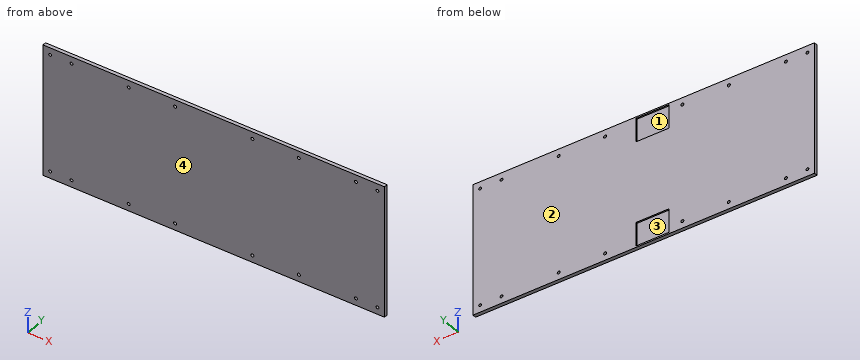
```python
from build123d import *

# Parameters (mm, degrees)
ESQUISSE1_W             = 478.153686012
ESQUISSE1_H             = 188.593708553
ESQUISSE1_R             = 2
BOSS_EXTRU_4_DEPTH      = 5
ESQUISSE2_W             = 35.2
ESQUISSE2_H             = 34
ESQUISSE2_W_2           = 11
ENL_V_MAT_EXTRU_1_DEPTH = 2
ESQUISSE3_R             = 2.1
ENL_V_MAT_EXTRU_2_DEPTH = 10


with BuildPart() as part:
    # Esquisse1 → Boss.-Extru.4 (new body)
    with BuildSketch(Plane(origin=(0, 0, 0), x_dir=(1, 0, 0), z_dir=(0, 1, 0))):
        with Locations((166.159297522, 47.085285911)):
            Rectangle(ESQUISSE1_W, ESQUISSE1_H)
        with Locations(Location((-62.917545484, 131.382140187, 0), (0, 0, 270))):
            Circle(ESQUISSE1_R, mode=Mode.SUBTRACT)
        with Locations(Location((-62.917545484, -37.211568366, 0), (0, 0, 270))):
            Circle(ESQUISSE1_R, mode=Mode.SUBTRACT)
        with Locations(Location((395.236140528, -37.211568366, 0), (0, 0, 270))):
            Circle(ESQUISSE1_R, mode=Mode.SUBTRACT)
        with Locations(Location((395.236140528, 131.382140187, 0), (0, 0, 270))):
            Circle(ESQUISSE1_R, mode=Mode.SUBTRACT)
        with Locations(Location((-32.917545484, -37.211568366, 0), (0, 0, 270))):
            Circle(ESQUISSE1_R, mode=Mode.SUBTRACT)
        with Locations(Location((-32.917545484, 131.382140187, 0), (0, 0, 270))):
            Circle(ESQUISSE1_R, mode=Mode.SUBTRACT)
        with Locations(Location((365.236140528, 131.382140187, 0), (0, 0, 270))):
            Circle(ESQUISSE1_R, mode=Mode.SUBTRACT)
        with Locations(Location((365.236140528, -37.211568366, 0), (0, 0, 270))):
            Circle(ESQUISSE1_R, mode=Mode.SUBTRACT)
    extrude(amount=BOSS_EXTRU_4_DEPTH)

    # Esquisse2 → Enlèv. mat.-Extru.1 (cut)
    with BuildSketch(Plane(origin=(0, 5, 0), x_dir=(1, 0, 0), z_dir=(0, 1, 0))):
        with Locations((148.559297522, 122.382140187)):
            Rectangle(ESQUISSE2_W, ESQUISSE2_H)
        with Locations((171.659297522, 122.382140187)):
            Rectangle(ESQUISSE2_W_2, ESQUISSE2_H)
        with Locations((148.559297522, -28.211568366)):
            Rectangle(ESQUISSE2_W, ESQUISSE2_H)
        with Locations((171.659297522, -28.211568366)):
            Rectangle(ESQUISSE2_W_2, ESQUISSE2_H)
    extrude(amount=-ENL_V_MAT_EXTRU_1_DEPTH, mode=Mode.SUBTRACT)

    # Esquisse3 → Enlèv. mat.-Extru.2 (cut)
    with BuildSketch(Plane(origin=(0, 5, 0), x_dir=(1, 0, 0), z_dir=(0, 1, 0))):
        with Locations(Location((47.082454516, 131.382140187, 0), (0, 0, 270))):
            Circle(ESQUISSE3_R)
        with Locations(Location((47.082454516, -37.211568366, 0), (0, 0, 270))):
            Circle(ESQUISSE3_R)
        with Locations(Location((285.236140528, 131.382140187, 0), (0, 0, 270))):
            Circle(ESQUISSE3_R)
        with Locations(Location((285.236140528, -37.211568366, 0), (0, 0, 270))):
            Circle(ESQUISSE3_R)
        with Locations(Location((220.236140528, 131.382140187, 0), (0, 0, 270))):
            Circle(ESQUISSE3_R)
        with Locations(Location((220.236140528, -37.211568366, 0), (0, 0, 270))):
            Circle(ESQUISSE3_R)
        with Locations(Location((112.082454516, 131.382140187, 0), (0, 0, 270))):
            Circle(ESQUISSE3_R)
        with Locations(Location((112.082454516, -37.211568366, 0), (0, 0, 270))):
            Circle(ESQUISSE3_R)
    extrude(amount=-ENL_V_MAT_EXTRU_2_DEPTH, mode=Mode.SUBTRACT)


solid = part.part
```
Part model, mm, in its own coordinate system. Face numbers are marked on the shaded views. A direction names the side the tool comes from. Round coordinates to 2 decimals unless told otherwise and drop trailing zeros. Write each loop counter-clockwise with the first axis right and the second up, starting at its lowest first coordinate (ties: lowest second). Pieces come first, ordered by that corner, then holes. Notation, with made-up numbers: (32.25, 10.25) -> (45.25, 10.25) arc R13 cw to (45.25, 21.25) -> close; hole circle Ø4 at (47.5, -22). An arc over 180 degrees is marked (long way). Return JSON: item names as keys, results as strings. Group by question number.
Q1. Pin check, flat tip, straight feed: pin 1 (5 mm diameter, centred on x = -62.92, z = -131.38, fed in from +Y). Stop position of the tip, or through.
Q2. Saw through at A-A on x = 138. Write the cut outline in (y, z).
Q3. Which spindle directions (+Z, -Z, +X, -X, +Y, -Y) get a long thin tool onto all of the face, cutting with end or side? Do the marked faces 3 and 4. Say none if no direction does.
Q4. Mould opens along Z. For the marked faces 1 and 2 say: pulls with the +Z half, pulls with the -Z half, needs draft (parallel to the pull), parting line crosses it, or undercut.
Q5. Probe L1, parallel to Z at x = 134.5, y = 4.75; L2, parallel to Z at x = -31.5, y = 2.8; L3, parallel to X at y = 4.7, z = 32.5. List the from-to ranges inside material, lowest first. Write a range as [from, to].
Q6. Saw through at B-B on z = -117. Write the cut outline in (x, y), plus the area to 3 significant figures.
Answer:
{
 "1": {"pin 1": "y = 5"},
 "2": {"outline": "(0, -141.38) -> (5, -141.38) -> (5, -139.38) -> (3, -139.38) -> (3, -105.38) -> (5, -105.38) -> (5, 11.21) -> (3, 11.21) -> (3, 45.21) -> (5, 45.21) -> (5, 47.21) -> (0, 47.21) -> close"},
 "3": {"face 3": "+Y", "face 4": "+Z, -Z, +X, -X, -Y"},
 "4": {"face 1": "undercut", "face 2": "needs draft"},
 "5": {"L1": "[-141.38, -139.38], [-105.38, 11.21], [45.21, 47.21]", "L2": "[-141.38, -132.79], [-129.97, 35.8], [38.62, 47.21]", "L3": "[-72.92, 130.96], [177.16, 405.24]"},
 "6": {"outline": "(-72.92, 0) -> (405.24, 0) -> (405.24, 5) -> (177.16, 5) -> (177.16, 3) -> (130.96, 3) -> (130.96, 5) -> (-72.92, 5) -> close", "area": "2,300 mm2"}
}
